Could you check a few things on this model? Use its own coordinates, in mm. Coordinates: 2 decimals unless noted, no trailing zeros. Order: outer loops, then holes, each group sorted by start corner. A loop starts at its lowest first (then second) coordinate and runs counter-clockwise, first axis right, second up. Notation, with made-up numbers: (7, 80.5) - (50, 80.5) arc R16 cw to (50, 98.5) - close; hole circle Ø6 at (38.5, 58). An arc over 180 degrees is marked (long way). Answer as CSV lines item,"result". Start each with the question number.
1. I need wall thicknesses on probe 1 along Y at (x, z) = (-141.5, -345); probe 2 along Z at (x, y) = (88.5, 54). Which ranges of each line are inside material? Lowest first, please.
2. I want a section at C-C, the plane x = 140.5. List the corners of the cut face in (y, z) for me.
3. I want a section at D-D, the plane z = 221. List the corners of the cut face in (x, y) for me.
4. I want a section at B-B, the plane y = 72. List the corners of the cut face in (x, z) for me.
5. For pin 1 (3 mm diameter, centred on x = 74, z = 255, fed in from +Y), with a flat end and sliding along its axis, tell me the tip position at first contact or that it passes through.
6. I want a section at A-A, the plane z = 387.5. List the corners of the cut face in (x, y) for me.
from build123d import *

# Parameters (mm, degrees)
SKETCH_1_W      = 334
SKETCH_1_H      = 800
EXTRUDE_1_DEPTH = 20
SKETCH_3_R      = 12.5
EXTRUDE_4_DEPTH = 100
FILLET_1_R      = 12.5


with BuildPart() as part:
    # Эскиз1 → Бобышка-Вытянуть1 (new body)
    with BuildSketch(Plane(origin=(0, 0, 0), x_dir=(1, 0, 0), z_dir=(0, 1, 0))):
        Rectangle(SKETCH_1_W, SKETCH_1_H)
    extrude(amount=-EXTRUDE_1_DEPTH)

    # Эскиз3 → Бобышка-Вытянуть4 (add)
    with BuildSketch(Plane(origin=(0, 0, 0), x_dir=(1, 0, 0), z_dir=(0, 1, 0))):
        with Locations(Location((-87.470406544, -387.5, 0), (0, 0, 270))):
            Circle(SKETCH_3_R)
        with Locations(Location((87.470406544, -387.5, 0), (0, 0, 270))):
            Circle(SKETCH_3_R)
    extrude(amount=EXTRUDE_4_DEPTH)

    # Скругление1
    fillet_1_edges = [part.edges().sort_by_distance(p)[0] for p in [
        (-87.470406544, 100, 375),
        (87.470406544, 100, 375),
    ]]
    fillet(fillet_1_edges, radius=FILLET_1_R)


solid = part.part
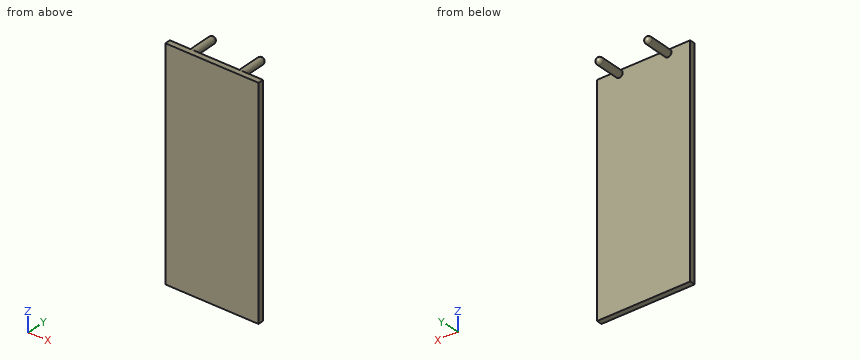
Solved:
1,probe 1,"y = -20 to 0"
1,probe 2,"z = 375.04 to 399.96"
2,outline,"(-20, -400) - (0, -400) - (0, 400) - (-20, 400) - close"
3,outline,"(-167, -20) - (167, -20) - (167, 0) - (-167, 0) - close"
4,outline,"circle Ø25 at (-87.47, 387.5); circle Ø25 at (87.47, 387.5)"
5,pin 1,"stops at y = 0"
6,outline,"(-167, -20) - (167, -20) - (167, 0) - (99.97, 0) - (99.97, 87.5) arc R12.5 ccw to (74.97, 87.5) - (74.97, 0) - (-74.97, 0) - (-74.97, 87.5) arc R12.5 ccw to (-99.97, 87.5) - (-99.97, 0) - (-167, 0) - close"
